The model under review builds one solid part; all positions refer to its coordinate system, in mm. Face numbers are marked on the shaded views. A direction names the side the tool comes from. Round coordinates to 2 decimals unless told otherwise and drop trailing zeros. Order: outer loops, then holes, each group sorted by start corner. A loop starts at its lowest first (then second) coordinate and runs counter-clockwise, first axis right, second up. Notation, with made-up numbers: M -7.75,2 L -1.75,2 A23 ccw -1.75,33 Z; hole C -29,53 d9. An arc over 180 degrees is marked long. Answer as a JSON object with one key per item and string values. Group by question number.
1. To check wall thickness, follow probe 1 along Y at (x, z) = (14.5, -6.75); probe 2 along Y at (x, z) = (-4.5, -3.25); probe 3 along Y at (x, z) = (-7, -3.5). State the ranges of each line that lie inside material, in increasing order. Write a range as [from, to].
2. Add section C-C on y = -8.25. State the section outline as (x, z) points.
3. Clearance check with flat-ended pins moving along their axes: P1, Ø3, axis at x = 10, y = -7, coming from the +Z side; P2, Ø8.5, axis at x = -6.5, y = -7, coming from the -Z side. State where each tip first meets the part, or that it passes through.
4. Add section A-A on z = -3.5. State the section outline as (x, y) points.
5. Add section D-D on x = -14. State the section outline as (y, z) points, and give its area (3 significant figures).
6. Machinability: for the marked faces 1 and 2, which of the approach directions +Z, -Z, +X, -X, +Y, -Y give a long, thin tool a straight path to every point of the face, cutting with its end or side? Answer none if there is none.
7. Mouldability with a two-part tool opening along Y and no side actions: class the marked faces 3, 4 and 5 as released by +Y, released by -Y, zero draft, split by the parting line, or undercut.
8. Add section B-B on z = -5.75. State the section outline as (x, y) points, and give its area (3 significant figures).
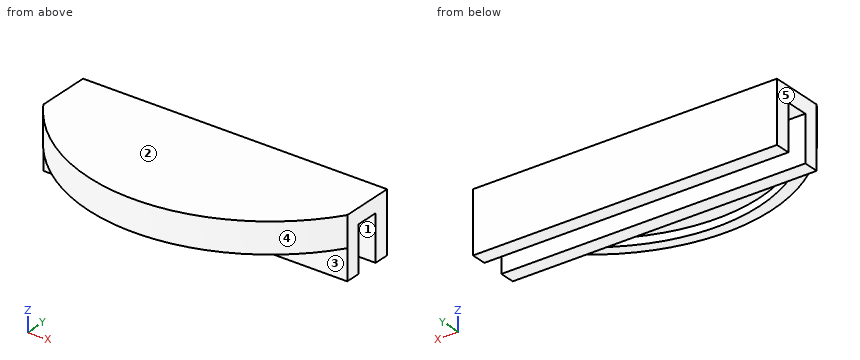
```python
from build123d import *

# Parameters (mm, degrees)
F0_W     = 40
F0_H     = 2
F1_DEPTH = 8
F2_DEPTH = 3
F4_DEPTH = 1
F5_W     = 40
F5_H     = 2
F6_DEPTH = 3
F7_W     = 40
F7_H     = 6
F7_H_2   = 2
F8_DEPTH = 2


with BuildPart() as f1:
    # F0 (on Top) → F1 (new body)
    with BuildSketch(Plane.XY):
        with Locations((0.387097, 1)):
            Rectangle(F0_W, F0_H)
    extrude(amount=-F1_DEPTH)

    # F0 (on Top) → F2 (join)
    with BuildSketch(Plane.XY):
        with BuildLine():
            Line((20.387097, 0), (-19.612903, 0))
            ThreePointArc((-19.612903, 0), (0.387097, -10.733501), (20.387097, 0))
        make_face()
    extrude(amount=-F2_DEPTH)

    # F3 (on face) → F4 (join)
    with BuildSketch(Plane(origin=(0, 0, -3), x_dir=(1, 0, 0), z_dir=(0, 0, -1))):
        with BuildLine():
            Line((18.387097, 0), (20.387097, 0))
            ThreePointArc((20.387097, 0), (0.387097, 10.733501), (-19.612903, 0))
            Line((-19.612903, 0), (-17.612903, 0))
            ThreePointArc((-17.612903, 0), (0.387097, 9.187189), (18.387097, 0))
        make_face()
    extrude(amount=F4_DEPTH)

    # F5 (on face) → F6 (join)
    with BuildSketch(Plane(origin=(0, 2, 0), x_dir=(-1, 0, 0), z_dir=(0, 1, 0))):
        with Locations((-0.387097, -1)):
            Rectangle(F5_W, F5_H)
    extrude(amount=F6_DEPTH)

    # F7 (on face) → F8 (join)
    with BuildSketch(Plane(origin=(0, 5, 0), x_dir=(-1, 0, 0), z_dir=(0, 1, 0))):
        with Locations((-0.387097, -5)):
            Rectangle(F7_W, F7_H)
        with Locations((-0.387097, -1)):
            Rectangle(F7_W, F7_H_2)
    extrude(amount=F8_DEPTH)


solid = f1.part
```
Recorded:
{
 "1": {"probe 1": "y = [0, 2], [5, 7]", "probe 2": "y = [-10.23, -8.64], [0, 2], [5, 7]", "probe 3": "y = [-9.57, -7.92], [0, 2], [5, 7]"},
 "2": {"outline": "M -10.24,-4 L -6,-4 L -6,-3 L 6.77,-3 L 6.77,-4 L 11.02,-4 L 11.02,0 L -10.24,0 Z"},
 "3": {"P1": "stops at z = 0", "P2": "stops at z = -4"},
 "4": {"outline": "M -19.61,0 A24 ccw 20.39,0 L 20.39,2 L -19.61,2 Z; M -19.61,5 L 20.39,5 L 20.39,7 L -19.61,7 Z; hole M -17.61,0 A22.23 ccw 18.39,0 Z"},
 "5": {"outline": "M -5.94,-4 L -3.9,-4 L -3.9,-3 L 0,-3 L 0,-8 L 2,-8 L 2,-2 L 5,-2 L 5,-8 L 7,-8 L 7,0 L -5.94,0 Z", "area": "57.9 mm²"},
 "6": {"face 1": "-Z, +X, -X", "face 2": "+Z, +X, -X, +Y, -Y"},
 "7": {"face 3": "undercut", "face 4": "released by -Y", "face 5": "zero draft"},
 "8": {"outline": "M -19.61,0 L 20.39,0 L 20.39,2 L -19.61,2 Z; M -19.61,5 L 20.39,5 L 20.39,7 L -19.61,7 Z", "area": "160 mm²"}
}
